Autodesk Inventor part; units mm, degrees
ref_plane "YZ Plane" through (0, 0, 0) normal (1, 0, 0) x (0, 1, 0)
ref_plane "XZ Plane" through (0, 0, 0) normal (0, 1, 0) x (-1, 0, 0)
ref_plane "XY Plane" through (0, 0, 0) normal (0, 0, 1) x (1, 0, 0)
sketch "Skizze1" plane through (0, 0, 0) normal (0, 1, 0) x (-1, 0, 0)
  line L0 (35.5112, -88.3128) -> (35.5112, -108.3128)
  line L1 (35.5112, -108.3128) -> (22.0645, -123.1178)
  line L2 (22.0645, -123.1178) -> (2.0645, -123.1178)
  line L3 (2.0645, -123.1178) -> (-12.7404, -109.6711)
  line L4 (-12.7404, -109.6711) -> (-12.7404, -89.6711)
  line L5 (-12.7404, -89.6711) -> (0.7063, -74.8661)
  line L6 (0.7063, -74.8661) -> (20.7063, -74.8661)
  line L7 (20.7063, -74.8661) -> (35.5112, -88.3128)
  point P0 (0, 0)
  dimension "d0" = 20
  dimension "d1" = 20
  dimension "d2" = 20
  dimension "d3" = 20
  dimension "d4" = 20
  dimension "d5" = 20
  dimension "d6" = 20
  dimension "d7" = 20
extrude "Extrusion1" add sketch "Skizze1" along normal blind 3
sketch "Skizze2" plane through (-2.0645, 0, -123.1178) normal (0, 0, -1) x (-1, 0, 0)
  circle A0 centre (10, 1.5) radius 2.5
  line L0 (0, 3) -> (20, 3)
  point P0 (-2.0645, 0)
  dimension "d11" = 5
  dimension "d12" = 1.5
extrude "Extrusion2" add sketch "Skizze2" along normal blind 81.748
sketch "Skizze3" plane through (-12.0645, 1.5, -204.8658) normal (0, 0, -1) x (-1, 0, 0)
  line L0 (-35, -15) -> (35, -15)
  line L1 (35, -15) -> (35, 15)
  line L2 (35, 15) -> (-35, 15)
  line L3 (-35, 15) -> (-35, -15)
  arc A0 (2, -1.5) -> (-2, -1.5) centre (0, 0) ccw
  line L4 (-35, -15) -> (35, 15) construction
  line L5 (35, -15) -> (-35, 15) construction
  point P0 (-12.0645, -1.5)
  point P1 (-2, 1.5)
  point P2 (0, -2.5)
  point P3 (0, 2.5)
  dimension "d15" = 70
  dimension "d16" = 30
extrude "Extrusion3" add sketch "Skizze3" against normal blind 2
sketch "Skizze6" plane through (-47.0645, -13.5, -204.8658) normal (0, -1, 0) x (1, 0, 0)
  line L0 (33, 81.748) -> (25, 81.748)
  line L1 (25, 81.748) -> (125.5267, 81.748)
  line L2 (125.5267, 81.748) -> (125.5267, -4.5987)
  line L3 (125.5267, -4.5987) -> (25, -4.5987)
  line L4 (25, -4.5987) -> (25, 81.748)
  line L5 (25, -4.5987) -> (-39.723, -4.5987)
  line L6 (-39.723, -4.5987) -> (-39.723, 43.9362)
  line L7 (-39.723, 43.9362) -> (25, 43.9362)
  line L8 (25, 43.9362) -> (25, -4.5987)
  point P0 (47.0645, 204.8658)
extrude "Extrusion5" cut sketch "Skizze6" against normal blind 50
properties part number "Stoppschild_Teil_Oben"
Design review of the part built by this model. Coordinates are the model's own, in mm. Coordinates: 2 decimals unless noted, no trailing zeros. Loops run counter-clockwise (first coordinate to the right, second up) from the corner with the lowest first, then second, coordinate; pieces in that order, holes last. Notation, with made-up numbers: (-36, -39) -> (-16, -39) arc R13 ccw to (-16, -20) -> close; hole circle Ø11 at (43, 10.25). An arc over 180 degrees is marked (long way). Use a Markdown table: item, result. Add a question column.
Item 1: We need section A-A, the plane y = 1.3. Write out the cut boundary in (x, z), and give its area (3 significant figures).
Item 2: We need section B-B, the plane z = -86.5. Write out the cut boundary in (x, y).
Item 3: Wall thickness on L1, parallel to X at y = 2.3, z = -115; L2, parallel to Z at x = -31, y = 0.3; L3, parallel to Z at x = -30, y = 0.9: over which ranges is each line inside the solid? List them lowest first. Write a range as from..to.
Item 4: We need section C-C, the plane x = 5. Write out the cut boundary in (y, z), and give its area (3 significant figures).
Numbers:
| question | item | result |
|---|---|---|
| 1 | outline | (-35.51, -108.31) -> (-22.06, -123.12) -> (-2.06, -123.12) -> (12.74, -109.67) -> (12.74, -89.67) -> (-0.71, -74.87) -> (-20.71, -74.87) -> (-35.51, -88.31) -> close |
| 1 | area | 1,930 mm^2 |
| 2 | outline | (-33.52, 0) -> (9.86, 0) -> (9.86, 3) -> (-33.52, 3) -> close |
| 3 | L1 | x = -29.44..6.87 |
| 3 | L2 | z = -113.28..-84.22 |
| 3 | L3 | z = -114.38..-83.31 |
| 4 | outline | (0, -116.7) -> (3, -116.7) -> (3, -81.15) -> (0, -81.15) -> close |
| 4 | area | 107 mm^2 |
